Check sheet for the modelled part. Datum: model origin and axes. Units: mm. Give positions to 0.01 mm unless a question says otherwise; leave off trailing zeros. Order: outer loops, then holes, each group sorted by start corner. A loop starts at its lowest first (then second) coordinate and runs counter-clockwise, first axis right, second up. Notation, with made-up numbers: (75.25, 63) - (89.25, 63) arc R16 cw to (89.25, 67) - close; hole circle Ø5 at (68.25, 28). An arc over 180 degrees is marked (long way). Answer in a Markdown table with one row per item.
from build123d import *

# Parameters (mm, degrees)
SKETCH_1_R                   = 45
EXTRUDE_1_DEPTH              = 3
HOLE_WIZARD_M3_1_D           = 2.5
HOLE_WIZARD_M3_1_CSINK_D     = 2.55
HOLE_WIZARD_M3_1_CSINK_ANGLE = 90
SKETCH_7_R                   = 1.5
SKETCH_7_W                   = 7.385
SKETCH_7_H                   = 2.7
SKETCH_7_W_2                 = 39.84
SKETCH_7_H_2                 = 20
CUT_EXTRUDE_1_DEPTH          = 4
CUT_EXTRUDE_1_DEPTH_BACK     = 1


with BuildPart() as part:
    # 草图1 → 凸台-拉伸1 (new body)
    with BuildSketch(Plane(origin=(0, 0, 0), x_dir=(1, 0, 0), z_dir=(0, 1, 0))):
        Circle(SKETCH_1_R)
    extrude(amount=EXTRUDE_1_DEPTH)

    # M3 螺纹孔的螺纹孔钻头1 (through all)
    with Locations(Plane.XZ):
        with Locations((40, 0), (12.360679775, 38.042260652), (-32.360679775, 23.511410092), (-32.360679775, -23.511410092), (12.360679775, -38.042260652)):
            CounterSinkHole(HOLE_WIZARD_M3_1_D / 2, HOLE_WIZARD_M3_1_CSINK_D / 2, counter_sink_angle=HOLE_WIZARD_M3_1_CSINK_ANGLE)

    # 草图7 → 切除-拉伸1 (cut, two sides)
    with BuildSketch(Plane(origin=(0, 0, 0), x_dir=(1, 0, 0), z_dir=(0, 1, 0))) as cut_extrude_1_sk:
        with Locations((14.53, 4.975)):
            Circle(SKETCH_7_R)
        with Locations((14.53, -4.975)):
            Circle(SKETCH_7_R)
        with Locations((-34.53, 4.975)):
            Circle(SKETCH_7_R)
        with Locations((-34.53, -4.975)):
            Circle(SKETCH_7_R)
        with Locations((13.6125, 0)):
            Rectangle(SKETCH_7_W, SKETCH_7_H)
        with Locations((-33.6125, 0)):
            Rectangle(SKETCH_7_W, SKETCH_7_H)
        with Locations((-10, 0)):
            Rectangle(SKETCH_7_W_2, SKETCH_7_H_2)
    extrude(amount=CUT_EXTRUDE_1_DEPTH, mode=Mode.SUBTRACT)
    extrude(cut_extrude_1_sk.sketch, amount=-CUT_EXTRUDE_1_DEPTH_BACK, mode=Mode.SUBTRACT)


solid = part.part
(1) Gauge pin test, flat ends, axial feed: P1, Ø0.9, axis at y = 1, z = 5, coming from the +X side; P2, Ø0.9, axis at x = -33.5, y = 2, coming from the -Z side. Record the tip position at first contact, or that the pin passes through.
Geometry says:
| item | result |
|---|---|
| P1 | x = 44.77 |
| P2 | z = -30.54 |
(2) Mould release check, pull along X, two halves, no side actions. Record for faces 1 (the cylindrical face through (20.765, 1.479, 39.923)), 2 (the cylindrical face through (13.03, 1.48, -5.04)), 3 (the flat face through (-1, 3, -11)): pulls with the +X half, pulls with the -X half, needs draft (parallel to the pull), parting line crosses it, or undercut.
Geometry says:
| item | result |
|---|---|
| face 1 | parting line crosses it |
| face 2 | undercut |
| face 3 | needs draft |
(3) Cross-section at B-B, the plane z = 0. Record the cut outline in (x, y) (3 decimals).
Geometry says:
| item | result |
|---|---|
| outline | (-45, 0) - (-37.305, 0) - (-37.305, 3) - (-45, 3) - close; (17.305, 0) - (38.725, 0) - (38.75, 0.025) - (38.75, 3) - (17.305, 3) - close; (41.25, 0.025) - (41.275, 0) - (45, 0) - (45, 3) - (41.25, 3) - close |
(4) Cross-section at A-A, the plane x = 0. Record the cut outline in (y, z), then the cut area to 3 significant figures.
Geometry says:
| item | result |
|---|---|
| outline | (0, -45) - (3, -45) - (3, -10) - (0, -10) - close; (0, 10) - (3, 10) - (3, 45) - (0, 45) - close |
| area | 210 mm² |
(5) Thickness scan on L1, parallel to X at y = 0.8, z = 0 (3 decimals); L2, parallel to Z at x = -34.53, y = 2.35 (3 decimals); L3, parallel to X at y = 1.4, z = 6. Record the ranges inside material, lowest first.
Geometry says:
| item | result |
|---|---|
| L1 | -45 to -37.305, 17.305 to 38.75, 41.25 to 45 |
| L2 | -28.856 to -6.475, -3.475 to -1.35, 1.35 to 3.475, 6.475 to 28.856 |
| L3 | -44.6 to -35.63, -33.43 to -29.92, 9.92 to 13.43, 15.63 to 44.6 |
(6) Cross-section at D-D, the plane x = 40. Record the cut outline in (y, z) (3 decimals).
Geometry says:
| item | result |
|---|---|
| outline | (0, -20.616) - (3, -20.616) - (3, -1.25) - (0.025, -1.25) - (0, -1.275) - close; (0, 1.275) - (0.025, 1.25) - (3, 1.25) - (3, 20.616) - (0, 20.616) - close |
(7) Cross-section at C-C, the plane y = 1.95. Give the number of separate pieces and of enclosed holes in the cut face, then the cut area to 3 significant figures.
Geometry says:
| item | result |
|---|---|
| separate pieces | 1 |
| enclosed holes | 10 |
| area | 5,470 mm² |
